from build123d import *

# Parameters (mm, degrees)
BOSS_EXTRUDE1_DEPTH          = 10
BOSS_EXTRUDE2_DEPTH          = 25
CUT_EXTRUDE_THIN1_DEPTH      = 77.865548199
CUT_EXTRUDE_THIN1_DEPTH_BACK = 19.5
SKETCH5_W                    = 9.5
SKETCH5_H                    = 83.5
CUT_EXTRUDE1_DEPTH           = 25
FILLET2_R                    = 1
SKETCH8_R                    = 3.25
CUT_EXTRUDE2_DEPTH           = 54
CUT_EXTRUDE3_DEPTH           = 30
BOSS_EXTRUDE5_START          = 2
BOSS_EXTRUDE5_DEPTH          = 2
BOSS_EXTRUDE6_DEPTH          = 1


with BuildPart() as part:
    # Sketch1 → Boss-Extrude1 (new body)
    with BuildSketch(Plane.XY):
        with BuildLine():
            Line((-4.75, -61.75), (4.75, -61.75))
            ThreePointArc((4.75, -61.75), (11.821067812, -58.821067812), (14.75, -51.75))
            Line((14.75, -51.75), (14.75, 51.75))
            ThreePointArc((14.75, 51.75), (11.821067812, 58.821067812), (4.75, 61.75))
            Line((4.75, 61.75), (-4.75, 61.75))
            ThreePointArc((-4.75, 61.75), (-11.821067812, 58.821067812), (-14.75, 51.75))
            Line((-14.75, 51.75), (-14.75, -51.75))
            ThreePointArc((-14.75, -51.75), (-11.821067812, -58.821067812), (-4.75, -61.75))
        make_face()
    extrude(amount=BOSS_EXTRUDE1_DEPTH)

    # Sketch3 → Boss-Extrude2 (add)
    with BuildSketch(Plane.XY.offset(10)):
        with BuildLine():
            Line((14.75, -51.75), (14.75, -21.75))
            Line((14.75, -21.75), (-14.75, -21.75))
            Line((-14.75, -21.75), (-14.75, -51.75))
            ThreePointArc((-14.75, -51.75), (-11.821067812, -58.821067812), (-4.75, -61.75))
            Line((-4.75, -61.75), (4.75, -61.75))
            ThreePointArc((4.75, -61.75), (11.821067812, -58.821067812), (14.75, -51.75))
        make_face()
    extrude(amount=BOSS_EXTRUDE2_DEPTH)

    # Sketch4 → Cut-Extrude-Thin1 (cut, two sides: drawn at the far end of the back side and taken through both)
    with BuildSketch(Plane(origin=(14.75, 0, 0), x_dir=(0, 0, -1), z_dir=(1, 0, 0)).offset(-CUT_EXTRUDE_THIN1_DEPTH_BACK)):
        Polygon((-34, -74.39853969), (-34, -25.75), (-30, -25.75), (-30, -57.75), (-24, -57.75), (-24, -25.75), (-20, -25.75), (-20, -57.75), (-18, -57.75), (-18, -23.75), (-26, -23.75), (-26, -55.75), (-28, -55.75), (-28, -23.75), (-36, -23.75), (-36, -74.39853969), align=None)
    extrude(amount=CUT_EXTRUDE_THIN1_DEPTH + CUT_EXTRUDE_THIN1_DEPTH_BACK, mode=Mode.SUBTRACT)

    # Sketch5 → Cut-Extrude1 (cut)
    with BuildSketch(Plane(origin=(0, 0, 0), x_dir=(-1, 0, 0), z_dir=(0, 0, -1))):
        with Locations((0, 20)):
            Rectangle(SKETCH5_W, SKETCH5_H)
    extrude(amount=-CUT_EXTRUDE1_DEPTH, mode=Mode.SUBTRACT)

    # Fillet2
    fillet2_edges = [part.edges().sort_by_distance(p)[0] for p in [
        (5, -25.75, 24),
        (4, -57.75, 30),
        (4, -57.75, 24),
        (5, -25.75, 20),
        (5, -23.75, 18),
        (5, -23.75, 28),
        (5, -23.75, 26),
        (4.582575695, -55.75, 26),
        (4.582575695, -55.75, 28),
        (5, -25.75, 30),
    ]]
    fillet(fillet2_edges, radius=FILLET2_R - 0.0001)  # a hair under: the kernel refuses the full size

    # Sketch8 → Cut-Extrude2 (cut)
    with BuildSketch(Plane(origin=(0, -21.75, 0), x_dir=(1, 0, 0), z_dir=(0, 1, 0))):
        with Locations(Location((0, -14, 0), (0, 0, 180))):
            Circle(SKETCH8_R)
    extrude(amount=-CUT_EXTRUDE2_DEPTH, mode=Mode.SUBTRACT)

    # Sketch9 → Cut-Extrude3 (cut)
    with BuildSketch(Plane(origin=(0, -61.75, 0), x_dir=(-1, 0, 0), z_dir=(0, -1, 0))):
        Polygon((0, -9.381197846), (-4, -11.690598923), (-4, -16.309401077), (0, -18.618802154), (4, -16.309401077), (4, -11.690598923), align=None)
    extrude(amount=-CUT_EXTRUDE3_DEPTH, mode=Mode.SUBTRACT)

    # Sketch11 → Boss-Extrude5 (add)
    with BuildSketch(Plane(origin=(0, 0, 0), x_dir=(-1, 0, 0), z_dir=(0, 0, -1)).offset(BOSS_EXTRUDE5_START)):
        with BuildLine():
            Line((-4.75, -66.75), (4.75, -66.75))
            ThreePointArc((4.75, -66.75), (15.356601718, -62.356601718), (19.75, -51.75))
            Line((19.75, -51.75), (19.75, 51.75))
            ThreePointArc((19.75, 51.75), (15.356601718, 62.356601718), (4.75, 66.75))
            Line((4.75, 66.75), (4.75, 61.75))
            ThreePointArc((4.75, 61.75), (11.821067812, 58.821067812), (14.75, 51.75))
            Line((14.75, 51.75), (14.75, -51.75))
            ThreePointArc((14.75, -51.75), (11.821067812, -58.821067812), (4.75, -61.75))
            Line((4.75, -61.75), (-4.75, -61.75))
            ThreePointArc((-4.75, -61.75), (-11.821067812, -58.821067812), (-14.75, -51.75))
            Line((-14.75, -51.75), (-14.75, 51.75))
            ThreePointArc((-14.75, 51.75), (-11.821067812, 58.821067812), (-4.75, 61.75))
            Line((-4.75, 61.75), (-4.75, 66.75))
            ThreePointArc((-4.75, 66.75), (-15.356601718, 62.356601718), (-19.75, 51.75))
            Line((-19.75, 51.75), (-19.75, -51.75))
            ThreePointArc((-19.75, -51.75), (-15.356601718, -62.356601718), (-4.75, -66.75))
        make_face()
        with BuildLine():
            ThreePointArc((14.75, 51.75), (11.821067812, 58.821067812), (4.75, 61.75))
            Line((4.75, 61.75), (4.75, -21.75))
            Line((4.75, -21.75), (-4.75, -21.75))
            Line((-4.75, -21.75), (-4.75, 61.75))
            ThreePointArc((-4.75, 61.75), (-11.821067812, 58.821067812), (-14.75, 51.75))
            Line((-14.75, 51.75), (-14.75, -51.75))
            ThreePointArc((-14.75, -51.75), (-11.821067812, -58.821067812), (-4.75, -61.75))
            Line((-4.75, -61.75), (4.75, -61.75))
            ThreePointArc((4.75, -61.75), (11.821067812, -58.821067812), (14.75, -51.75))
            Line((14.75, -51.75), (14.75, 51.75))
        make_face()
    extrude(amount=-BOSS_EXTRUDE5_DEPTH)

    # Sketch12 → Boss-Extrude6 (add)
    with BuildSketch(Plane.XY.offset(34)):
        with BuildLine():
            Line((5, -25.75), (4.75, -61.75))
            ThreePointArc((4.75, -61.75), (11.821067812, -58.821067812), (14.75, -51.75))
            Line((14.75, -51.75), (14.75, -25.75))
            Line((14.75, -25.75), (5, -25.75))
        make_face()
    extrude(amount=BOSS_EXTRUDE6_DEPTH)


solid = part.part
Design review of the part built by this model. Coordinates are the model's own, in mm. A direction names the side the tool comes from. Coordinates: 2 decimals unless noted, no trailing zeros. Loops run counter-clockwise (first coordinate to the right, second up) from the corner with the lowest first, then second, coordinate; pieces in that order, holes last. Notation, with made-up numbers: (-4.75, 89.25) -> (33.25, 89.25) arc R34 cw to (33.25, 121.25) -> close; hole circle Ø7 at (59, 69.5). An arc over 180 degrees is marked (long way). Use a Markdown table: item, result. Add a question column.
Item 1: Wall thickness on L1, parallel to Z at x = 10.5, y = -27; L2, parallel to Z at x = 11, y = -56; L3, parallel to Z at x = 0, y = -28: over which ranges is each line inside the solid? List them lowest first. Write a range as from..to.
Item 2: We need section C-C, the plane z = 5. Write out the cut boundary in (x, y).
Item 3: We need section D-D, the plane x = -8.5. Write out the cut boundary in (y, z), and give its area (3 significant figures).
Item 4: The part is to be moulded in two halves that separate along Y. For faces 1 (the cylindrical face through (-15.47, 62.24, -1.01)), 2 (the flat face through (5, -42, 30)), 3 (the flat face through (10, 21, 10)), say which applies: +Y half, -Y half, draft (parallel to the pull), parting line (faces both ways), or undercut.
Item 5: Machinability: for faces 4 (the flat face through (0, -61.75, 21)), 5 (the cylindrical face through (11.9, 58.74, 4.93)), 6 (the flat face through (4, -57.75, 27)), 7 (the flat face through (5, -25.75, 33)), 8 (the flat face through (4.75, 22, 4)), which of the approach directions +Z, -Z, +X, -X, +Y, -Y give a long, thin tool a straight path to every point of the face, cutting with its end or side? Answer none if there is none.
Item 6: Clearance check with flat-ended pins moving along their axes: P1, Ø6.5, axis at x = 3, z = 30.5, coming from the -Y side; P2, Ø4.5, axis at y = -40, z = 22, coming from the +X side; P3, Ø3, axis at x = -9, z = 22, coming from the +Y side; P4, Ø8, axis at x = 1, y = -26.5, coming from the +Z side. State where each tip first meets the part, or that it passes through.
Item 7: We need section A-A, the plane z = 14. Write out the cut boundary in (x, y).
Item 8: We need section B-B, the plane y = -16. Write out the cut boundary in (x, z).
Numbers:
| question | item | result |
|---|---|---|
| 1 | L1 | z = -2..18, 20..24, 26..28, 30..35 |
| 1 | L2 | z = -2..18, 20..24, 30..35 |
| 1 | L3 | z = -2..10.75, 17.25..18, 20..24, 26..28, 30..34 |
| 2 | outline | (-14.75, -51.75) arc R10 ccw to (-4.75, -61.75) -> (4.75, -61.75) arc R10 ccw to (14.75, -51.75) -> (14.75, 51.75) arc R10 ccw to (4.75, 61.75) -> (4.75, -21.75) -> (-4.75, -21.75) -> (-4.75, 61.75) arc R10 ccw to (-14.75, 51.75) -> close |
| 3 | outline | (-66.27, -2) -> (66.27, -2) -> (66.27, 0) -> (61.02, 0) -> (61.02, 10) -> (-21.75, 10) -> (-21.75, 35) -> (-61.02, 35) -> (-61.02, 0) -> (-66.27, 0) -> close |
| 3 | area | 2,470 mm^2 |
| 4 | face 1 | +Y half |
| 4 | face 2 | undercut |
| 4 | face 3 | draft |
| 5 | face 4 | +Z, +X, -X, -Y |
| 5 | face 5 | +Z, +X, +Y |
| 5 | face 6 | +X |
| 5 | face 7 | +Z, +X |
| 5 | face 8 | +Z, -Z, +Y |
| 6 | P1 | stops at y = -61.75 |
| 6 | P2 | stops at x = 14.75 |
| 6 | P3 | stops at y = -21.75 |
| 6 | P4 | stops at z = 35 |
| 7 | outline | (-14.75, -51.75) arc R10 ccw to (-4.75, -61.75) -> (-4, -61.75) -> (-4, -31.75) -> (-3.25, -31.75) -> (-3.25, -21.75) -> (-14.75, -21.75) -> close; (3.25, -31.75) -> (4, -31.75) -> (4, -61.75) -> (4.75, -61.75) arc R10 ccw to (14.75, -51.75) -> (14.75, -21.75) -> (3.25, -21.75) -> close |
| 8 | outline | (-19.75, -2) -> (-4.75, -2) -> (-4.75, 10) -> (-14.75, 10) -> (-14.75, 0) -> (-19.75, 0) -> close; (4.75, -2) -> (19.75, -2) -> (19.75, 0) -> (14.75, 0) -> (14.75, 10) -> (4.75, 10) -> close |
